Here's the drawing with two shaded views (mm, measured from the low corner). I have some questions. Round coordinates to 2 decimals unless told otherwise and drop trailing zeros. Order: outer loops, then holes, each group sorted by start corner. A loop starts at its lowest first (then second) coordinate and runs counter-clockwise, first axis right, second up. Notation, with made-up numbers: (-27, 45.25) - (8, 45.25) arc R29 ccw to (8, 84.25) - close; hole circle Ø6 at (-35.75, 43). An arc over 180 degrees is marked (long way). One line per item, written item: value.
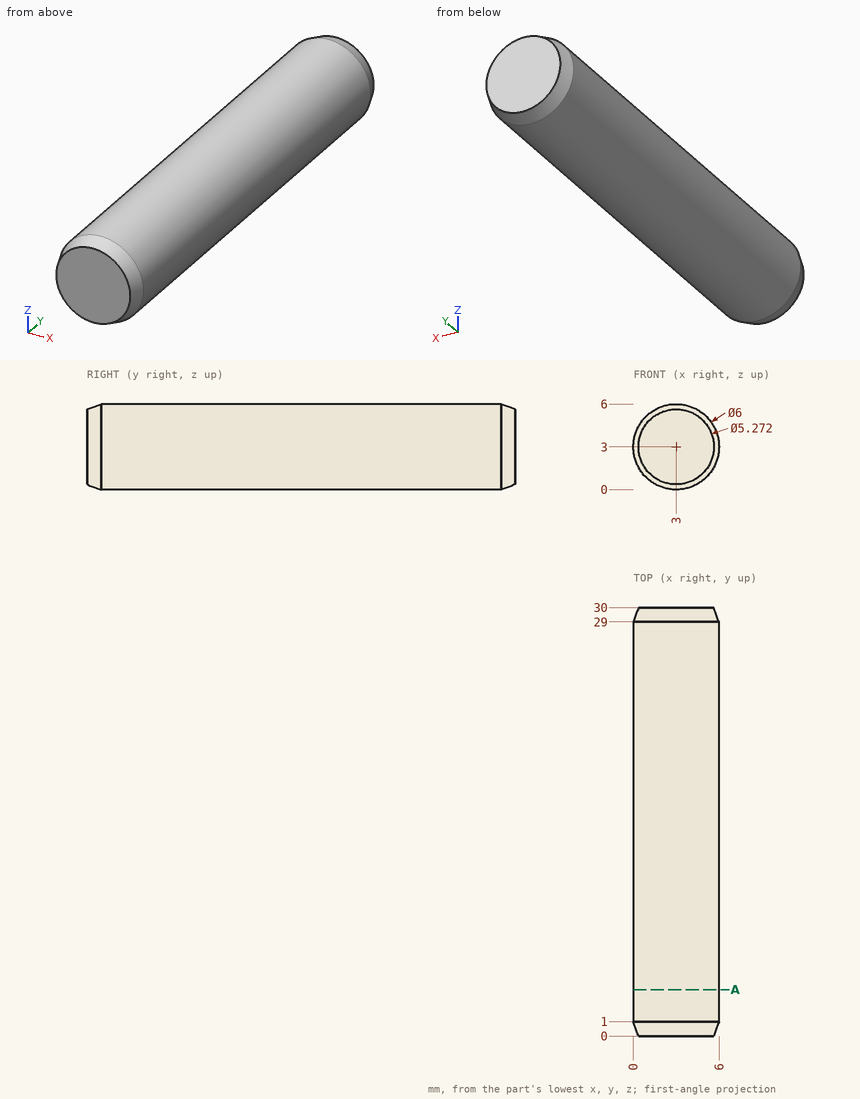
Q1. If I drill on line 1 along X through (y, z) = (18.5, 3.9); line 2 along X through (y, z) = (15, 4.25); line 3 along Z through (x, y) = (3.15, 5.25), over which ranges is the centre line in solid material (lowest first)?
Results list:
line 1: 0.14 to 5.86
line 2: 0.27 to 5.73
line 3: 0 to 6
Q2. Will this pin go through, and if not, where does the flat tip stop? pin 1 (2 mm diameter, centred on x = 4.5, y = 19, fed in from -Z).
Results list:
pin 1: z = 0.04
Q3. If we section it at A-A, the plane y = 3.25: Please give me the cut outline in (x, z).
Results list:
outline: circle Ø6 at (3, 3)
